```python
from build123d import *

# Parameters (mm, degrees)
F0_W      = 51.88
F0_H      = 114.8
F1_DEPTH  = 9.28
F2_R      = 5
F3_T      = -2.5
F4_W      = 9.99
F4_H      = 3.45
F5_DEPTH  = 69.5
F6_W      = 21.96
F6_H      = 2.88
F7_DEPTH  = 36.6
F8_W      = 44.31
F8_H      = 5.84
F9_DEPTH  = 65.7
F10_R     = 16.320489
F11_DEPTH = 1.2


with BuildPart() as f1:
    # F0 (on Top) → F1 (new body)
    with BuildSketch(Plane.XY):
        with Locations((-0.042248, -0.113639)):
            Rectangle(F0_W, F0_H)
    extrude(amount=F1_DEPTH)

    # F2
    f2_edges = [f1.edges().sort_by_distance(p)[0] for p in [
        (25.897752, 57.286361, 4.64),
        (25.897752, -57.513639, 4.64),
        (-25.982248, 57.286361, 4.64),
        (-25.982248, -57.513639, 4.64),
    ]]
    fillet(f2_edges, radius=F2_R)

    # F3
    f3_openings = [f1.faces().sort_by_distance(p)[0] for p in [
        (-0.042248, -0.113639, 9.28),
    ]]
    offset(amount=F3_T, openings=f3_openings)

    # F4 (on Front) → F5 (cut)
    with BuildSketch(Plane.XZ):
        with Locations((-14.695825, 4.658578)):
            Rectangle(F4_W, F4_H)
    extrude(amount=F5_DEPTH, mode=Mode.SUBTRACT)

    # F6 (on Right) → F7 (cut)
    with BuildSketch(Plane.YZ):
        with Locations((-36.337859, 4.790666)):
            Rectangle(F6_W, F6_H)
    extrude(amount=F7_DEPTH, mode=Mode.SUBTRACT)

    # F8 (on Front) → F9 (cut)
    with BuildSketch(Plane.XZ):
        with Locations((-1.091603, 4.939306)):
            Rectangle(F8_W, F8_H)
    extrude(amount=-F9_DEPTH, mode=Mode.SUBTRACT)

    # F10 (on Top) → F11 (join)
    with BuildSketch(Plane.XY):
        with BuildLine():
            ThreePointArc((18.784328, -6.925963), (19.709026, -3.517707), (20.020488, 0))
            ThreePointArc((20.020488, 0), (19.709026, 3.517707), (18.784328, 6.925963))
            ThreePointArc((18.784328, 6.925963), (0, 20.020488), (-18.784328, 6.925963))
            ThreePointArc((-18.784328, 6.925963), (-20.020488, 0), (-18.784328, -6.925963))
            ThreePointArc((-18.784328, -6.925963), (0, -20.020488), (18.784328, -6.925963))
        make_face()
        Circle(F10_R, mode=Mode.SUBTRACT)
        with BuildLine():
            ThreePointArc((-18.784328, 6.925963), (0, 20.020488), (18.784328, 6.925963))
            Line((18.784328, 6.925963), (22.793854, 6.925963))
            Line((22.793854, 6.925963), (22.793854, 42.115439))
            Line((22.793854, 42.115439), (0, 42.115439))
            Line((0, 42.115439), (-22.793854, 42.115439))
            Line((-22.793854, 42.115439), (-22.793854, 6.925963))
            Line((-22.793854, 6.925963), (-18.784328, 6.925963))
        make_face()
        with BuildLine():
            Line((22.793854, -6.925963), (18.784328, -6.925963))
            ThreePointArc((18.784328, -6.925963), (0, -20.020488), (-18.784328, -6.925963))
            Line((-18.784328, -6.925963), (-22.793854, -6.925963))
            Line((-22.793854, -6.925963), (-22.793854, -42.115439))
            Line((-22.793854, -42.115439), (0, -42.115439))
            Line((0, -42.115439), (22.793854, -42.115439))
            Line((22.793854, -42.115439), (22.793854, -6.925963))
        make_face()
    extrude(amount=-F11_DEPTH)


solid = f1.part
```
Verification items for the finished model (mm, model axes). A direction names the side the tool comes from. Give positions to 0.01 mm unless a question says otherwise; leave off trailing zeros. Loops run counter-clockwise (first coordinate to the right, second up) from the corner with the lowest first, then second, coordinate; pieces in that order, holes last.
1. Go/stop test with flat-tipped pins: pin 1 Ø10 at (x, y) = (-15.5, -30) entering from +Z; pin 2 Ø1.3 at (x, z) = (20, -1) entering from +Y; pin 3 Ø3 at (y, z) = (-33, 6) entering from +X; pin 4 Ø4 at (x, y) = (-2.5, 6) entering from +Z. Record where each tip stops, or that it passes through.
2. Mould release check, pull along Y, two halves, no side actions. Record for faces 1 (the flat face through (0, 57.286, 1)), 2 (the cylindrical face through (22.646, -54.301, 5.937)), 3 (the flat face through (-25, -4, 9.28)): released by +Y, released by -Y, zero draft, split by the parting line, or undercut.
3. Section check C-C, the plane y = -32. Enter the section's corners in (x, z), then the cut area to 3 significant figures.
4. Section check B-B, the plane x = 0. Enter the section's corners in (y, z).
5. Thickness scan on line 1 (X direction, y = -32.5, z = 7); line 2 (Y direction, x = 0, z = -0.4); line 3 (Y direction, x = 13.5, z = 6.5). Record the ranges inside material, lowest first.
6. Section check D-D, the plane y = 29. Enter the section's corners in (x, z).
7. Set-up check for faces 4 (the flat face through (25, -25.358, 5)), 5 (the flat face through (21.063, 37, 2.3)), 6 (the cylindrical face through (-3.54, -15.93, -0.59)), 7 (the flat face through (-19.691, -56, 5)), 8 (the cylindrical face through (-22.77, -54.26, 5.94)): record each of +Z, -Z, +X, -X, +Y, -Y from which the full face is reachable in a straight line by a thin tool's end or side.
8. Section check A-A, the plane x = -17.5. Enter the section's corners in (y, z), then the cut area to 3 significant figures.
Geometry says:
1. pin 1: stops at z = 2.5
1. pin 2: stops at y = 42.12
1. pin 3: stops at x = 25.9
1. pin 4: stops at z = 2.02
2. face 1: released by +Y
2. face 2: undercut
2. face 3: zero draft
3. outline: (-25.98, 0) - (-22.79, 0) - (-22.79, -1.2) - (22.79, -1.2) - (22.79, 0) - (25.9, 0) - (25.9, 3.35) - (23.4, 3.35) - (23.4, 2.5) - (-23.48, 2.5) - (-23.48, 9.28) - (-25.98, 9.28) - close; (23.4, 6.23) - (25.9, 6.23) - (25.9, 9.28) - (23.4, 9.28) - close
3. area: 211 mm2
4. outline: (-57.51, 0) - (-42.12, 0) - (-42.12, -1.2) - (-16.32, -1.2) - (-16.32, 0) - (16.32, 0) - (16.32, -1.2) - (42.12, -1.2) - (42.12, 0) - (57.29, 0) - (57.29, 2.02) - (0, 2.02) - (0, 2.5) - (-55.01, 2.5) - (-55.01, 9.28) - (-57.51, 9.28) - close; (54.79, 7.86) - (57.29, 7.86) - (57.29, 9.28) - (54.79, 9.28) - close
5. line 1: x = -25.98 to -23.48, 23.4 to 25.9
5. line 2: y = -42.12 to -16.32, 16.32 to 42.12
5. line 3: y = -57.51 to -55.01
6. outline: (-25.98, 0) - (-22.79, 0) - (-22.79, -1.2) - (22.79, -1.2) - (22.79, 0) - (25.9, 0) - (25.9, 9.28) - (23.4, 9.28) - (23.4, 2.5) - (21.06, 2.5) - (21.06, 2.02) - (-23.25, 2.02) - (-23.25, 2.5) - (-23.48, 2.5) - (-23.48, 9.28) - (-25.98, 9.28) - close
7. face 4: +X
7. face 5: +Y
7. face 6: -Z
7. face 7: +Y, -Y
7. face 8: +Z
8. outline: (-57.51, 0) - (-42.12, 0) - (-42.12, -1.2) - (42.12, -1.2) - (42.12, 0) - (57.29, 0) - (57.29, 2.02) - (0, 2.02) - (0, 2.5) - (-55.01, 2.5) - (-55.01, 2.93) - (-57.51, 2.93) - close; (-57.51, 6.38) - (-55.01, 6.38) - (-55.01, 9.28) - (-57.51, 9.28) - close; (54.79, 7.86) - (57.29, 7.86) - (57.29, 9.28) - (54.79, 9.28) - close
8. area: 372 mm2
